Design review of the part shown in the three views and the two pictorial views. Dimensions are in mm from the part's minimum x, y and z. Round coordinates to 2 decimals unless told otherwise and drop trailing zeros. Loops run counter-clockwise (first coordinate to the right, second up) from the corner with the lowest first, then second, coordinate; pieces in that order, holes last.
1) Insertion check: pin 1 (2.5 mm diameter, centred on y = 249.5, z = 2.5, fed in from -X); pin 2 (2.5 mm diameter, centred on x = 243.5, y = 103.9, fed in from -Z); pin 3 (3 mm diameter, centred on x = 241, z = 0.5, fed in from -Y); pin 4 (1 mm diameter, centred on x = 179, z = 4, fed in from +Y). Each pin has a flat end and moves straight along its axis. Give the tip position at first contact, or say it passes through.
2) Take a section at C-C (z = 1.4). Give the number of separate pieces and of enclosed holes in the cut face, then the cut area to 3 significant figures.
3) Wall thickness on L1, parallel to Y at x = 243.5, z = 3; L2, parallel to X at y = 74.1, z = 1.15; L3, parallel to Y at x = 67, z = 3.55: over which ranges is each line inside the solid? List them lowest first.
4) Take a section at B-B (x = 43). State the section outline as (y, z) points.
5) Take a section at A-A (y = 258). State the section outline as (x, z) points, then the cut area to 3 significant figures.
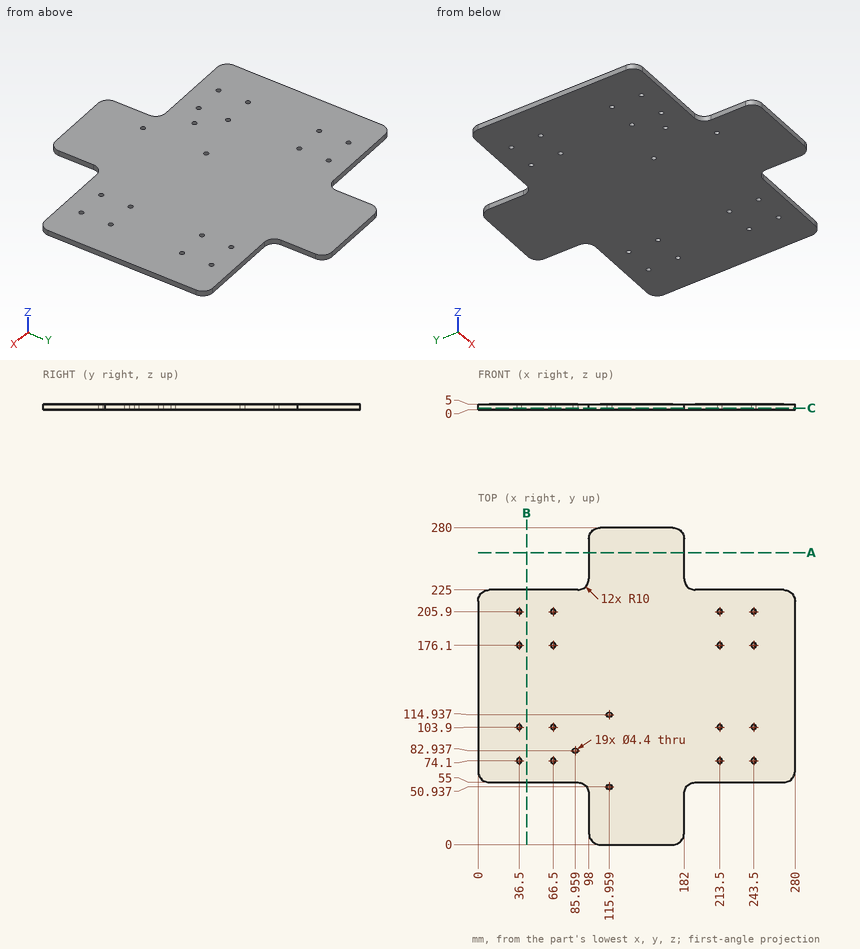
Response:
1. pin 1: stops at x = 98
1. pin 2: passes through
1. pin 3: stops at y = 55
1. pin 4: stops at y = 277.6
2. separate pieces: 1
2. enclosed holes: 19
2. area: 56,500 mm2
3. L1: y = 55 to 71.9, 76.3 to 101.7, 106.1 to 173.9, 178.3 to 203.7, 208.1 to 225
3. L2: x = 0 to 34.3, 38.7 to 64.3, 68.7 to 211.3, 215.7 to 241.3, 245.7 to 280
3. L3: y = 55 to 71.96, 76.24 to 101.76, 106.04 to 173.96, 178.24 to 203.76, 208.04 to 225
4. outline: (55, 0) - (225, 0) - (225, 5) - (55, 5) - close
5. outline: (98, 0) - (182, 0) - (182, 5) - (98, 5) - close
5. area: 420 mm2
